Read the model definition and answer for the solid it produces. Units are mm, in the model's axes. Coordinates: 2 decimals unless noted, no trailing zeros. Order: outer loops, then holes, each group sorted by start corner. A loop starts at its lowest first (then second) coordinate and runs counter-clockwise, first axis right, second up. Notation, with made-up numbers: (34.5, 53.5) - (84.5, 53.5) arc R24 cw to (84.5, 76.5) - close; hole circle Ø7 at (13, 51.25). An arc over 180 degrees is marked (long way). Write item = value, one per line.
Solid Edge part; units mm, degrees
sketch "Sketch1" plane through (0, 0, -32) normal (0, 0, -1) x (-1, 0, 0)
  circle A0 centre (-117.75, 0) radius 35.5
  circle A1 centre (-117.75, 0) radius 9.5
extrude "Protrusion1" add sketch "Sketch1" along normal blind 5
chamfer "Faza_1" distance 0.5 angle 45 2 edges at (127.25, 0, -37) (153.25, 0, -37)
hole "Otwór_1" at (138.6097, -20.8597, -37) direction (0, 0, 1) diameter 6.647 end up to next start chamfer 0.6 start chamfer angle 45 end chamfer 0.6 end chamfer angle 45
hole "Hole1" at (117.75, -29.5, -37) direction (0, 0, 1) diameter 6.647 end up to next start chamfer 0.6 start chamfer angle 45 end chamfer 0.6 end chamfer angle 45
hole "Hole2" at (96.8903, -20.8597, -37) direction (0, 0, 1) diameter 6.647 end up to next start chamfer 0.6 start chamfer angle 45 end chamfer 0.6 end chamfer angle 45
hole "Hole3" at (96.8903, 20.8597, -37) direction (0, 0, 1) diameter 6.647 end up to next start chamfer 0.6 start chamfer angle 45 end chamfer 0.6 end chamfer angle 45
hole "Hole4" at (117.75, 29.5, -37) direction (0, 0, 1) diameter 6.647 end up to next start chamfer 0.6 start chamfer angle 45 end chamfer 0.6 end chamfer angle 45
hole "Hole5" at (138.6097, 20.8597, -37) direction (0, 0, 1) diameter 6.647 end up to next start chamfer 0.6 start chamfer angle 45 end chamfer 0.6 end chamfer angle 45
1) Flat-ended cylindrical pins translate along their axes: pin 1 Ø1.5 at (y, z) = (-13, -36) entering from -X; pin 2 Ø10.5 at (x, y) = (117.75, -29.5) entering from +Z; pin 3 Ø2 at (x, z) = (121, -36) entering from -Y; pin 4 Ø2 at (x, z) = (122, -35) entering from +Y. Find the tip coordinate at first contact, or state that the pin passes through.
Returned:
pin_1 = 84.43
pin_2 = -32
pin_3 = -35.43
pin_4 = 35.35
2) The part is cut by section B-B (x = 117.75). Determine the outline of the cut face in (y, z).
Returned:
outline = (-35.5, -36.5) - (-35, -37) - (-33.42, -37) - (-32.82, -36.4) - (-32.82, -32.6) - (-33.42, -32) - (-35.5, -32) - close; (-26.18, -36.4) - (-25.58, -37) - (-10, -37) - (-9.5, -36.5) - (-9.5, -32) - (-25.58, -32) - (-26.18, -32.6) - close; (9.5, -36.5) - (10, -37) - (25.58, -37) - (26.18, -36.4) - (26.18, -32.6) - (25.58, -32) - (9.5, -32) - close; (32.82, -36.4) - (33.42, -37) - (35, -37) - (35.5, -36.5) - (35.5, -32) - (33.42, -32) - (32.82, -32.6) - close
3) The part is cut by section C-C (z = -35.5). Determine the outline of the cut face in (x, y).
Returned:
outline = circle Ø71 at (117.75, 0); hole circle Ø6.65 at (96.89, -20.86); hole circle Ø6.65 at (96.89, 20.86); hole circle Ø19 at (117.75, 0); hole circle Ø6.65 at (117.75, -29.5); hole circle Ø6.65 at (117.75, 29.5); hole circle Ø6.65 at (138.61, -20.86); hole circle Ø6.65 at (138.61, 20.86)
4) The part is cut by section D-D (x = 98). Count the separate pieces of the cut face and the enclosed holes in it, and give its area (3 significant figures).
Returned:
separate_pieces = 3
enclosed_holes = 0
area = 231 mm^2
5) The part is cut by section A-A (y = 0). Determine the outline of the cut face in (x, z).
Returned:
outline = (82.25, -36.5) - (82.75, -37) - (107.75, -37) - (108.25, -36.5) - (108.25, -32) - (82.25, -32) - close; (127.25, -36.5) - (127.75, -37) - (152.75, -37) - (153.25, -36.5) - (153.25, -32) - (127.25, -32) - close
6) Straight lines are drawn through the part: line 1 along Y through (x, z) = (117.75, -34.85); line 2 along Y through (x, z) = (96, -36.1); line 3 along Y through (x, z) = (94.5, -34.8). For each, find the intervals that lie inside material, in ascending order. Write a range as from..to.
Returned:
line_1 = -35.5..-32.82, -26.18..-9.5, 9.5..26.18, 32.82..35.5
line_2 = -28.06..-24.06, -17.66..17.66, 24.06..28.06
line_3 = -26.83..-23.17, -18.55..18.55, 23.17..26.83
7) Determine the mould class of faces 1 (the face through (145.92, 21.6, -34.22)), 2 (the face through (110, -7, -32)), 3 (the face through (108.689, -2.854, -34.218)) for opening direction X: pulls with the +X half, pulls with the -X half, needs draft (parallel to the pull), parting line crosses it, or undercut.
Returned:
face_1 = parting line crosses it
face_2 = needs draft
face_3 = undercut
